The listing builds one solid part. Answer for the finished solid, in the listing's coordinates (mm). Face numbers are marked on the shaded views. A direction names the side the tool comes from. Give positions to 0.01 mm unless a question says otherwise; leave off trailing zeros. Write each loop counter-clockwise with the first axis right and the second up, starting at its lowest first coordinate (ties: lowest second). Pieces come first, ordered by that corner, then holes. Notation, with made-up numbers: (88, 71) -> (114, 71) arc R20 ccw to (114, 103) -> close; hole circle Ø4 at (-37.5, -2). An arc over 180 degrees is marked (long way). Use CSV: the item, a comma, the result in double quotes. Start each with the question number.
Autodesk Fusion 360 part; units mm, degrees
sketch "Sketch1" plane through (0, 0, 0) normal (0, 0, 1) x (1, 0, 0)
  line L0 (21.15, -21.15) -> (-21.15, -21.15)
  line L1 (-21.15, -21.15) -> (-21.15, 21.15)
  line L2 (-21.15, 21.15) -> (21.15, 21.15)
  line L3 (21.15, 21.15) -> (21.15, -21.15)
  line L4 (21.15, -21.15) -> (-21.15, 21.15) construction
  line L5 (-21.15, -21.15) -> (21.15, 21.15) construction
  line L6 (-8.1, -21.15) -> (8.1, -21.15)
  line L7 (-8.1, -21.15) -> (-8.1, -31.15)
  line L8 (-8.1, -31.15) -> (8.1, -31.15)
  line L9 (8.1, -31.15) -> (8.1, -21.15)
  line L10 (15.5, 15.5) -> (-15.5, 15.5) construction
  line L11 (-15.5, 15.5) -> (-15.5, -15.5) construction
  line L12 (-15.5, -15.5) -> (15.5, -15.5) construction
  line L13 (15.5, -15.5) -> (15.5, 15.5) construction
  line L14 (15.5, 15.5) -> (-15.5, -15.5) construction
  line L15 (-15.5, 15.5) -> (15.5, -15.5) construction
  circle A0 centre (-15.5, -15.5) radius 3
  circle A1 centre (15.5, -15.5) radius 3
  line L16 (1.75, 0) -> (22.5, 0)
  circle A2 centre (15.5, 15.5) radius 3
  circle A3 centre (-15.5, 15.5) radius 3
  dimension "d1" = 42.3
  dimension "d2" = 42.3
  dimension "d5" = 10
  dimension "d6" = 16.2
  dimension "d7" = 13.05
  dimension "d23" = 31
  dimension "d24" = 31
  dimension "d25" = 6
  dimension "d26" = 6
extrude "Extrude1" add sketch "Sketch1" along normal blind 38 contours L0 L1 L2 L3 L6 | A0 | A1 | A2 | A3
extrude "Extrude2" add sketch "Sketch1" along normal blind 9.4 contours L0 L6 L7 L8 L9
sketch "Sketch2" plane through (0, 0, 38) normal (0, 0, 1) x (-1, 0, 0)
  line L0 (21.15, 21.15) -> (-21.15, 21.15)
  line L1 (-21.15, 21.15) -> (-21.15, -21.15)
  line L2 (-21.15, -21.15) -> (21.15, -21.15)
  line L3 (21.15, -21.15) -> (21.15, 21.15)
  circle A0 centre (0, 0) radius 2.5
  dimension "d12" = 5
extrude "Extrude3" add sketch "Sketch2" along normal blind 23.9 contours A0
sketch "Sketch3" plane through (0, 0, 38) normal (0, 0, 1) x (-1, 0, 0)
  circle A0 centre (0, 0) radius 2.5
  line L0 (21.15, 21.15) -> (-21.15, 21.15)
  line L1 (-21.15, 21.15) -> (-21.15, -21.15)
  line L2 (-21.15, -21.15) -> (21.15, -21.15)
  line L3 (21.15, -21.15) -> (21.15, 21.15)
  line L4 (-15.5, 15.5) -> (15.5, 15.5) construction
  line L5 (15.5, 15.5) -> (15.5, -15.5) construction
  line L6 (15.5, -15.5) -> (-15.5, -15.5) construction
  line L7 (-15.5, -15.5) -> (-15.5, 15.5) construction
  line L8 (-15.5, 15.5) -> (15.5, -15.5) construction
  line L9 (15.5, 15.5) -> (-15.5, -15.5) construction
  circle A1 centre (15.5, -15.5) radius 1.5
  circle A2 centre (-15.5, -15.5) radius 1.5
  circle A3 centre (-15.5, 15.5) radius 1.5
  circle A4 centre (15.5, 15.5) radius 1.5
  circle A5 centre (0, 0) radius 11
  dimension "d15" = 31
  dimension "d16" = 31
  dimension "d17" = 3
  dimension "d18" = 3
  dimension "d19" = 3
  dimension "d20" = 3
  dimension "d30" = 22
extrude "Extrude4" cut sketch "Sketch3" against normal up to surface (38 mm away) contours A1 | A2 | A3 | A4
extrude "Extrude5" cut sketch "Sketch1" along normal blind 3 contours A0 | A1 | A2 | A3
chamfer "Chamfer1" distance 1.5 angle 45 4 edges at (12.703, -16.5848, 3) (-18.297, -16.5848, 3) (12.703, 14.4152, 3) (-18.297, 14.4152, 3)
extrude "Extrude6" add sketch "Sketch3" along normal blind 2.2 contours A5
sketch "Sketch4" plane through (0, 0, 61.9) normal (0, 0, 1) x (-1, 0, 0)
  circle A0 centre (0, 0) radius 2.5
  line L0 (0, 0) -> (2.25, 0)
  line L1 (2.25, 0) -> (2.25, -2.5)
  line L2 (2.25, -2.5) -> (2.25, 0)
  line L3 (2.25, 0) -> (2.25, 2.5)
  dimension "d34" = 2.25
extrude "Extrude7" cut sketch "Sketch4" against normal blind 18 contours A0 L1 L2 L3 picked at (2.4114, -0.0938)
chamfer "Chamfer3" distance 0.5 angle 45 1 edges at (10.2556, -3.9778, 38)
sketch "Sketch5" plane through (0, -31.15, 0) normal (0, -1, 0) x (1, 0, 0)
  line L0 (-8.1, 0) -> (8.1, 0)
  line L1 (8.1, 0) -> (8.1, 9.4)
  line L2 (8.1, 9.4) -> (-8.1, 9.4)
  line L3 (-8.1, 9.4) -> (-8.1, 0)
  line L4 (-8.1, 0) -> (-8.1, 2.6)
  line L5 (-8.1, 2.6) -> (8.1, 2.6)
  line L6 (8.1, 2.6) -> (8.1, 0)
  line L7 (8.1, 0) -> (-8.1, 0)
  line L8 (8.1, 2.6) -> (8.1, 9.4)
  line L9 (8.1, 9.4) -> (4.5, 9.4)
  line L10 (-8.1, 2.6) -> (-8.1, 9.4)
  line L11 (-8.1, 9.4) -> (-4.5, 9.4)
  line L12 (-7.6, 8.9) -> (-4.5, 8.9)
  line L13 (-7.6, 3.1) -> (-7.6, 8.9)
  line L14 (-7.6, 3.1) -> (7.6, 3.1)
  line L15 (7.6, 3.1) -> (7.6, 8.9)
  line L16 (7.6, 8.9) -> (4.5, 8.9)
  line L17 (-4.5, 8.9) -> (-4.5, 9.4)
  line L18 (4.5, 9.4) -> (4.5, 8.9)
  dimension "d38" = 2.6
  dimension "d39" = 3.6
  dimension "d40" = -0.5
extrude "Extrude8" cut sketch "Sketch5" against normal up to surface (10 mm away) contours L2 L12 L13 L14 L15 L16 L17 L18
extrude "Extrude9" add sketch "Sketch5" along normal blind 0.5 contours L1 L2 L3 L5 L8 L9 L10 L11 L12 L13 L14 L15 L16 L17 L18
sketch "Sketch6" plane through (0, -21.15, 0) normal (0, -1, 0) x (1, 0, 0)
  line L0 (21.15, 38) -> (-21.15, 38)
  line L1 (8.1, 0) -> (21.15, 0)
  line L2 (-8.1, 0) -> (-8.1, 9.4)
  line L3 (-8.1, 9.4) -> (-4.5, 9.4)
  line L4 (-4.5, 9.4) -> (-4.5, 8.9)
  line L5 (-4.5, 8.9) -> (-7.6, 8.9)
  line L6 (-7.6, 8.9) -> (-7.6, 3.1)
  line L7 (-7.6, 3.1) -> (7.6, 3.1)
  line L8 (7.6, 3.1) -> (7.6, 8.9)
  line L9 (7.6, 8.9) -> (4.5, 8.9)
  line L10 (4.5, 8.9) -> (4.5, 9.4)
  line L11 (4.5, 9.4) -> (8.1, 9.4)
  line L12 (8.1, 9.4) -> (8.1, 0)
  line L13 (7.6, 3.1) -> (7.6, 8.9)
  line L14 (7.6, 6) -> (6.6, 6) construction
  line L15 (6.6, 6) -> (0, 6) construction
  line L16 (0, 6) -> (3.3, 6) construction
  line L17 (3.3, 6) -> (6.6, 6) construction
  circle A0 centre (6.6, 6) radius 0.25
  line L18 (0, 6) -> (1, 6)
  line L19 (1, 6) -> (6.6, 6) construction
  circle A1 centre (4.125, 6) radius 0.25
  circle A2 centre (1.65, 6) radius 0.25
  line L20 (0, 6) -> (0, 5.2231)
  circle A3 centre (-4.125, 6) radius 0.25
  circle A4 centre (-6.6, 6) radius 0.25
  circle A5 centre (-1.65, 6) radius 0.25
  line L21 (21.15, 0) -> (21.15, 38)
  line L22 (-21.15, 38) -> (-21.15, 0)
  line L23 (-21.15, 0) -> (-8.1, 0)
  dimension "d45" = 1
  dimension "d46" = 0.5
  dimension "d48" = 1
  dimension "d49" = 0.5
  dimension "d50" = 0.5
  dimension "d51" = 2.475
  dimension "d52" = 2.475
extrude "Extrude10" add sketch "Sketch6" along normal up to surface (10.5 mm away) contours A0 | A1 | A2 | A3 | A4 | A5
sketch "Sketch7" plane through (0, 21.15, 0) normal (0, 1, 0) x (-1, 0, 0)
  line L0 (-21.15, 0) -> (21.15, 0)
  line L1 (21.15, 0) -> (21.15, 38)
  line L2 (21.15, 38) -> (-21.15, 38)
  line L3 (-21.15, 38) -> (-21.15, 0)
  line L4 (0, 0) -> (0, 8) construction
  line L5 (0, 8) -> (-21.15, 8)
  line L6 (-21.15, 8) -> (-21.15, 0)
  line L7 (0, 8) -> (21.15, 8)
  line L8 (21.15, 8) -> (21.15, 0)
  line L9 (0, 0) -> (0, 38) construction
  line L10 (0, 19) -> (2, 19)
  line L11 (0, 38) -> (0, 30) construction
  line L12 (0, 30) -> (21.15, 30)
  line L13 (21.15, 30) -> (21.15, 38)
  line L14 (0, 30) -> (-21.15, 30)
  line L15 (-21.15, 30) -> (-21.15, 38)
  dimension "d55" = 8
  dimension "d56" = 8
extrude "Extrude11" add sketch "Sketch7" along normal blind 0.01 contours L0 L1 L3 L5 L6 L7 L8 | L1 L2 L3 L12 L13 L14 L15
sketch "Sketch8" plane through (0, -21.15, 0) normal (0, -1, 0) x (1, 0, 0)
  circle A0 centre (-6.6, 6) radius 0.25
  circle A1 centre (4.125, 6) radius 0.25
  circle A2 centre (1.65, 6) radius 0.25
  circle A3 centre (-4.125, 6) radius 0.25
  circle A4 centre (6.6, 6) radius 0.25
  circle A5 centre (-1.65, 6) radius 0.25
  line L0 (-8.1, 0) -> (-8.1, 9.4)
  line L1 (-8.1, 9.4) -> (-4.5, 9.4)
  line L2 (-4.5, 9.4) -> (-4.5, 8.9)
  line L3 (-4.5, 8.9) -> (-7.6, 8.9)
  line L4 (-7.6, 8.9) -> (-7.6, 3.1)
  line L5 (-7.6, 3.1) -> (7.6, 3.1)
  line L6 (7.6, 3.1) -> (7.6, 8.9)
  line L7 (7.6, 8.9) -> (4.5, 8.9)
  line L8 (4.5, 8.9) -> (4.5, 9.4)
  line L9 (4.5, 9.4) -> (8.1, 9.4)
  line L10 (8.1, 9.4) -> (8.1, 0)
  line L11 (8.1, 0) -> (21.15, 0)
  line L12 (21.15, 0) -> (21.15, 38)
  line L13 (21.15, 38) -> (-21.15, 38)
  line L14 (-21.15, 38) -> (-21.15, 0)
  line L15 (-21.15, 0) -> (-8.1, 0)
  line L16 (-21.15, 38) -> (-21.15, 30)
  line L17 (-21.15, 30) -> (21.15, 30)
  line L18 (21.15, 30) -> (21.15, 38)
  line L19 (0, 38) -> (0, 0) construction
  line L20 (0, 0) -> (0, 19) construction
  line L21 (2.7667, 19) -> (0, 19)
  line L22 (-21.15, 0) -> (-21.15, 8)
  line L23 (21.15, 8) -> (21.15, 0)
  line L24 (-21.15, 8) -> (21.15, 8)
  dimension "d59" = 8
  dimension "d60" = 8
extrude "Extrude12" add sketch "Sketch8" along normal blind 0.01 contours L0 L14 L15 L22 L24 | L12 L13 L14 L16 L17 L18 | L10 L11 L12 L23 L24
sketch "Sketch9" plane through (21.15, 0, 0) normal (1, 0, 0) x (0, 1, 0)
  line L0 (-21.16, 0) -> (21.16, 0)
  line L1 (21.16, 0) -> (21.16, 8)
  line L2 (21.16, 8) -> (21.15, 8)
  line L3 (21.15, 8) -> (21.15, 30)
  line L4 (21.15, 30) -> (21.16, 30)
  line L5 (21.16, 30) -> (21.16, 38)
  line L6 (21.16, 38) -> (-21.16, 38)
  line L7 (-21.16, 38) -> (-21.16, 30)
  line L8 (-21.16, 30) -> (-21.15, 30)
  line L9 (-21.15, 30) -> (-21.15, 8)
  line L10 (-21.15, 8) -> (-21.16, 8)
  line L11 (-21.16, 8) -> (-21.16, 0)
  line L12 (21.16, 30) -> (-21.16, 30)
  line L13 (-21.16, 8) -> (21.15, 8)
sketch "Sketch10" plane through (-21.15, 0, 0) normal (-1, 0, 0) x (0, -1, 0)
  line L0 (-21.16, 0) -> (21.16, 0)
  line L1 (21.16, 0) -> (21.16, 8)
  line L2 (21.16, 8) -> (21.15, 8)
  line L3 (21.15, 8) -> (21.15, 30)
  line L4 (21.15, 30) -> (21.16, 30)
  line L5 (21.16, 30) -> (21.16, 38)
  line L6 (21.16, 38) -> (-21.16, 38)
  line L7 (-21.16, 38) -> (-21.16, 30)
  line L8 (-21.16, 30) -> (-21.15, 30)
  line L9 (-21.15, 30) -> (-21.15, 8)
  line L10 (-21.15, 8) -> (-21.16, 8)
  line L11 (-21.16, 8) -> (-21.16, 0)
  line L12 (21.15, 30) -> (-21.16, 30)
  line L13 (-21.15, 8) -> (21.16, 8)
extrude "Extrude13" cut sketch "Sketch10" against normal blind 0.01 contours L3 L9 L12 L13
extrude "Extrude14" cut sketch "Sketch9" against normal blind 0.01 contours L3 L9 L12 L13
chamfer "Chamfer4" distance 7 angle 45 1 edges at (-21.14, -21.15, 19)
chamfer "Chamfer5" distance 7 angle 45 3 edges at (21.14, -21.15, 19) (21.14, 21.15, 19) (-21.14, 21.15, 19)
chamfer "Chamfer6" distance 5.5 angle 45 8 edges at (-21.15, 21.16, 4) (-21.15, -21.16, 4) (-21.15, -21.16, 34) (-21.15, 21.16, 34) (21.15, 21.16, 4) (21.15, -21.16, 4) (21.15, -21.16, 34) (21.15, 21.16, 34)
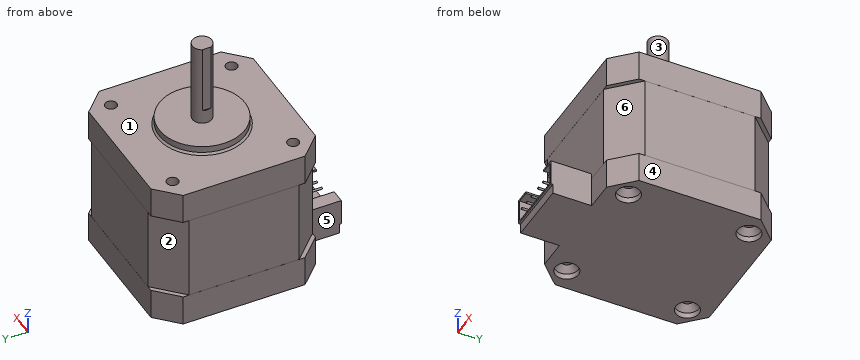
Q1. The mould has two halves that part along Z. Classify the marked faces 1, 2 and 3: +Z half, -Z half, draft (parallel to the pull), parting line (faces both ways), or undercut.
Q2. For the marked faces 4, 5 and 6, determine the directions among +Z, -Z, +X, -X, +Y, -Y from which every point of the face is accessible in a straight line to the end or side of a thin tool.
Q3. Straight lines are drawn through the part: L1, parallel to Y at x = 15.5, z = 0.9; L2, parallel to Y at x = 15.5, z = 30.5; L3, parallel to X at y = 16, z = 35.5. For each, find the intervals that lie inside material, in ascending order.
Q4. Flat-ended cylindrical pins translate along their axes: pin 1 Ø6 at (x, z) = (7, 38.5) entering from -Y; pin 2 Ø12.5 at (x, y) = (-6, -1) entering from +Z; pin 3 Ø4.5 at (y, z) = (-28.5, 7) entering from +X; pin 4 Ø10.5 at (y, z) = (-25.5, 7) entering from -X. Find the tip coordinate at first contact, or state that the pin passes through.
Q5. Section A-A on y = -22.5 is taken. Give the vertices of the cut face in (x, z) (3 decimals).
Output:
1,face 1,"+Z half"
1,face 2,"undercut"
1,face 3,"draft"
2,face 4,"+Z, -Z, +X, +Y, -Y"
2,face 5,"+Z, -Z, -X, -Y"
2,face 6,"+X, -Y"
3,L1,"-21.16 to -18.5, -12.5 to 12.5, 18.5 to 21.16"
3,L2,"-21.16 to -17, -14 to 14, 17 to 21.16"
3,L3,"-20.81 to -16.91, -14.09 to 14.09, 16.91 to 20.81"
4,pin 1,"y = -21.16"
4,pin 2,"z = 61.9"
4,pin 3,"x = 8.1"
4,pin 4,"x = -16.56"
5,outline,"(-8.1, 0) -> (8.1, 0) -> (8.1, 9.4) -> (4.5, 9.4) -> (4.5, 8.9) -> (7.6, 8.9) -> (7.6, 3.1) -> (-7.6, 3.1) -> (-7.6, 8.9) -> (-4.5, 8.9) -> (-4.5, 9.4) -> (-8.1, 9.4) -> close; circle Ø0.5 at (-6.6, 6); circle Ø0.5 at (-4.125, 6); circle Ø0.5 at (-1.65, 6); circle Ø0.5 at (1.65, 6); circle Ø0.5 at (4.125, 6); circle Ø0.5 at (6.6, 6)"
